```python
from build123d import *
from build123d.topology import SkipClean

# Parameters (mm, degrees)
EXTRUDE_1_DEPTH     = 2.5
SKETCH_3_R          = 10.25
SKETCH_3_R_2        = 1.55
CUT_EXTRUDE_1_DEPTH = 2.5
SKETCH_2_R          = 20.25
EXTRUDE_2_DEPTH     = 15
SKETCH_4_R          = 1.5
CUT_EXTRUDE_2_DEPTH = 46.33118669
CUT_EXTRUDE_3_DEPTH = 11


with BuildPart() as part:
    # Эскиз1 → Бобышка-Вытянуть1 (new body)
    with BuildSketch(Plane(origin=(0, 0, 0), x_dir=(0, 0, -1), z_dir=(1, 0, 0))):
        with BuildLine():
            Line((-30.866648668, -21.5), (0, -21.5))
            ThreePointArc((0, -21.5), (18.960941325, 10.135714286), (-17.877458963, 11.943469388))
            Line((-17.877458963, 11.943469388), (-35.024197264, -13.72244898))
            ThreePointArc((-35.024197264, -13.72244898), (-35.276169906, -18.857142857), (-30.866648668, -21.5))
        make_face()
    extrude(amount=EXTRUDE_1_DEPTH)

    # Эскиз3 → Вырез-Вытянуть1 (cut)
    with BuildSketch(Plane(origin=(2.5, 0, 0), x_dir=(0, 0, -1), z_dir=(1, 0, 0))):
        Circle(SKETCH_3_R)
        with Locations((3.882285677, 14.488887394)):
            Circle(SKETCH_3_R_2)
        with Locations((10.606601718, -10.606601718)):
            Circle(SKETCH_3_R_2)
        with Locations((-14.488887394, -3.882285677)):
            Circle(SKETCH_3_R_2)
    extrude(amount=-CUT_EXTRUDE_1_DEPTH, mode=Mode.SUBTRACT)

    # Эскиз2 → Бобышка-Вытянуть2 (add)
    with SkipClean():  # the faces are left unmerged after this step: merging them gives an invalid solid
        with BuildSketch(Plane.ZY.offset(-2.5)):
            with BuildLine():
                Line((0, -21.5), (30.866648668, -21.5))
                ThreePointArc((30.866648668, -21.5), (35.276169906, -18.857142857), (35.024197264, -13.72244898))
                Line((35.024197264, -13.72244898), (17.877458963, 11.943469388))
                ThreePointArc((17.877458963, 11.943469388), (-18.960941325, 10.135714286), (0, -21.5))
            make_face()
            Circle(SKETCH_2_R, mode=Mode.SUBTRACT)
        extrude(amount=-EXTRUDE_2_DEPTH)

    # Эскиз4 → Вырез-Вытянуть2 (cut, through all)
    with SkipClean():  # the faces are left unmerged after this step: merging them gives an invalid solid
        with BuildSketch(Plane(origin=(17.5, 0, 0), x_dir=(0, 0, -1), z_dir=(1, 0, 0))):
            with Locations((-30.866648668, -16.5)):
                Circle(SKETCH_4_R)
        extrude(amount=-CUT_EXTRUDE_2_DEPTH, mode=Mode.SUBTRACT)

    # Эскиз5 → Вырез-Вытянуть3 (cut)
    with SkipClean():  # the faces are left unmerged after this step: merging them gives an invalid solid
        with BuildSketch(Plane(origin=(17.5, 0, 0), x_dir=(0, 0, -1), z_dir=(1, 0, 0))):
            Polygon((-20.25, 4.5), (-19.743669872, 4.5), (-19.743669872, -4.5), (-20.25, -4.5), (-21.25, -4.5), (-21.25, 4.5), align=None)
        extrude(amount=-CUT_EXTRUDE_3_DEPTH, mode=Mode.SUBTRACT)


solid = part.part
```
The model under review builds one solid part; all positions refer to its coordinate system, in mm. A direction names the side the tool comes from. Round coordinates to 2 decimals unless told otherwise and drop trailing zeros. Write each loop counter-clockwise with the first axis right and the second up, starting at its lowest first coordinate (ties: lowest second). Pieces come first, ordered by that corner, then holes. Notation, with made-up numbers: M 0.5,25.5 L 13.5,25.5 A31 cw 13.5,54.5 Z; hole C -15.75,2 d3. An arc over 180 degrees is marked long. Use CSV: the item, a comma, the result in double quotes. Start each with the question number.
(1) Clearance check with flat-ended pins moving along their axes: P1, Ø3, axis at x = 9, y = 5, coming from the +Z side; P2, Ø1, axis at x = 9, y = 11, coming from the -Z side; P3, Ø2.5, axis at x = 11.5, y = -1.5, coming from the -Z side. State where each tip first meets the part, or that it passes through.
(2) We need section C-C, the plane z = -11. State the section outline as (x, y) points, then the cut area to 3 significant figures.
(3) For line 1 along Z through (x, y) = (12.75, -17.5); line 2 along Y through (x, z) = (6.5, 0); line 3 along X through (y, z) = (8, -13), list the stretches that pass through material, from the lowest coordinate up.
(4) The part is to be moulded in two halves that separate along Y. For faces 1 (the face through (17.5, -13, 18)), 2 (the face through (1.27, -10.54, -9.06)), 3 (the face through (1.268, 16.026, -3.681)), say which applies: +Y half, -Y half, draft (parallel to the pull), parting line (faces both ways), or undercut.
(5) We need section B-B, the plane y = -16.5. State the section outline as (x, z) points.
(6) We need section A-A, the plane x = 7.5. State the section outline as (y, z) points, then the cut area to 3 significant figures.
(7) We need section D-D, the plane x = 1.75. State the section outline as (y, z) points.
(8) Tool access review of faces 4 (the face through (1.268, -10.006, 2.222)), 5 (the face through (10, 17, 11)): name each direction out of +Z, -Z, +X, -X, +Y, -Y from which nothing blocks a thin tool from reaching the whole face with its end or side.
Findings:
1,P1,"z = 23.52"
1,P2,"z = -18.76"
1,P3,"z = -21.5"
2,outline,"M 0,-18.47 L 17.5,-18.47 L 17.5,-17 L 2.5,-17 L 2.5,-12.11 L 0,-12.11 Z; M 0,-9.11 L 2.5,-9.11 L 2.5,17 L 17.5,17 L 17.5,18.47 L 0,18.47 Z"
2,area,"129 mm^2"
3,line 1,"-12.49 to -10.19, 10.19 to 29.75, 31.98 to 35.77"
3,line 2,"-21.5 to -20.25, 20.25 to 21.5"
3,line 3,"0 to 2.5"
4,face 1,"draft"
4,face 2,"undercut"
4,face 3,"undercut"
5,outline,"M 0,-13.78 L 17.5,-13.78 L 17.5,-11.74 L 2.5,-11.74 L 2.5,11.74 L 17.5,11.74 L 17.5,29.37 L 0,29.37 Z; M 0,32.37 L 17.5,32.37 L 17.5,35.87 L 0,35.87 Z"
6,outline,"M -21.5,0 A21.5 ccw long 11.94,17.88 L -13.72,35.02 A5 ccw -21.5,30.87 Z; hole C -16.5,30.87 d3; hole M -4.5,19.74 A20.25 ccw long 4.5,19.74 L 4.5,21.25 L -4.5,21.25 Z"
6,area,"492 mm^2"
7,outline,"M -21.5,0 A21.5 ccw long 11.94,17.88 L -13.72,35.02 A5 ccw -21.5,30.87 Z; hole C -16.5,30.87 d3; hole C -10.61,-10.61 d3.1; hole C 0,0 d20.5; hole C -3.88,14.49 d3.1; hole C 14.49,-3.88 d3.1"
8,face 4,"+X, -X"
8,face 5,"+X"
